Design review of the part built by this model. Coordinates are the model's own, in mm. A direction names the side the tool comes from. Coordinates: 2 decimals unless noted, no trailing zeros. Loops run counter-clockwise (first coordinate to the right, second up) from the corner with the lowest first, then second, coordinate; pieces in that order, holes last. Notation, with made-up numbers: (70.25, -22.75) -> (125.25, -22.75) arc R16 cw to (125.25, -10.75) -> close; hole circle Ø11 at (52.5, -7). An arc over 180 degrees is marked (long way). Use a Markdown table: item, result. Add a question column.
Q1. Take a section at B-B on z = -9.5. Write out the cut boundary in (x, y), plus the area to 3 significant figures.
Q2. Take a section at D-D on z = -13. Write out the cut boundary in (x, y).
Q3. For faces 1 (the face through (-5, 6, -32)), 2 (the face through (-10, 5.9, -11.5)), 3 (the face through (-16.1, 11.5, -4)), 4 (the face through (-29.08, 11.49, -2.45)), 5 (the face through (-15, 1, -7)), list the 3-axis set-ups (+Z, -Z, +X, -X, +Y, -Y) from which the entire face can be reached by the end or side of a thin tool; tool diameter is ignored.
Q4. For probe 1 along X at (y, z) = (11.6, -5); probe 2 along Y at (x, z) = (-17.5, -8); probe 3 along Z at (x, y) = (-26, 0.5), list the stretches that pass through material, from the lowest coordinate up.
Q5. Clearance check with flat-ended pins moving along their axes: pin 1 Ø2 at (x, z) = (-7.5, -7) entering from -Y; pin 2 Ø0.5 at (y, z) = (7.5, -11.5) entering from -X; pin 3 Ø3 at (x, z) = (-26, -5) entering from -Y; pin 4 Ø1 at (y, z) = (4.5, -27) entering from +X. State where each tip first meets the part, or that it passes through.
Q6. Take a section at C-C on x = -15.5. Write out the cut boundary in (y, z), plus the area to 3 significant figures.
Q7. Draft analysis for pull direction Z (two halves, no side actions). For faces 6 (the face through (-16.1, 0.5, -4)), 7 (the face through (-17.888, 11.493, -10.014)), 8 (the face through (-27.6, 11.5, -6.2)), state which applies: pulls with the +Z half, pulls with the -Z half, needs draft (parallel to the pull), parting line crosses it, or undercut.
Q8. Take a section at A-A on x = -5. Write out the cut boundary in (y, z), plus the area to 3 significant figures.
Autodesk Inventor part; units mm, degrees
ref_plane "YZ Plane" through (0, 0, 0) normal (1, 0, 0) x (0, 1, 0)
ref_plane "XZ Plane" through (0, 0, 0) normal (0, 1, 0) x (-1, 0, 0)
ref_plane "XY Plane" through (0, 0, 0) normal (0, 0, 1) x (1, 0, 0)
sketch "Sketch1" plane through (0, 0, 0) normal (0, 1, 0) x (-1, 0, 0)
  line L0 (0, -12) -> (10, -12)
  line L1 (10, -12) -> (10, -5)
  line L2 (0, -5) -> (0, -12)
  arc A0 (10, -5) -> (0, -5) centre (5, -5) ccw
  circle A1 centre (5, -5) radius 2
  circle A2 centre (26, -5) radius 2
  line L3 (10, -4) -> (22, -4)
  line L4 (10, -12) -> (10, -11)
  line L5 (26, -9) -> (10, -11)
  arc A3 (26, -9) -> (22, -5) centre (26, -5) ccw
  line L6 (10, -4) -> (9.899, -4)
  line L7 (22, -4) -> (22.127, -4)
  point P0 (0, 0)
  point P1 (0, 0)
  point P2 (9.9495, -4)
  point P3 (5, 0)
  dimension "d269" = 4
  dimension "d270" = 12
  dimension "d271" = 1
  dimension "d272" = 4
  dimension "d273" = 4
  dimension "d274" = -1
  dimension "d275" = -1
  dimension "d278" = 7
  dimension "d279" = 10
  dimension "d280" = 5
  dimension "d282" = 4
  dimension "d284" = 5
  dimension "d286" = 5
  dimension "d287" = 4
extrude "Extrusion1" add sketch "Sketch1" along normal blind 1
sketch "Sketch2" plane through (0, 1, 0) normal (0, 1, 0) x (1, 0, 0)
  line L0 (0, 12) -> (-10, 12)
  line L1 (0, 12) -> (-10, 12)
  line L2 (-10, 12) -> (-10, 11)
  line L3 (-10, 11) -> (0, 11)
  line L4 (0, 11) -> (0, 12)
  point P0 (0, 0)
  dimension "d288" = 1
extrude "Extrusion2" add sketch "Sketch2" along normal blind 10
sketch "Sketch3" plane through (0, 11, 0) normal (0, 1, 0) x (1, 0, 0)
  line L0 (0, 5) -> (0, 12)
  line L1 (0, 12) -> (-10, 12)
  line L2 (-10, 12) -> (-10, 11)
  line L3 (0, 11) -> (0, 12)
  arc A0 (-9.899, 4) -> (0, 5) centre (-5, 5) ccw
  line L4 (0, 11) -> (0, 5)
  line L5 (-22.127, 4) -> (-9.899, 4)
  arc A1 (-9.899, 4) -> (0, 5) centre (-5, 5) ccw
  arc A2 (-26, 9) -> (-22.127, 4) centre (-26, 5) ccw
  line L6 (-9.899, 4) -> (-22.127, 4)
  line L7 (-10, 11) -> (-26, 9)
  line L8 (-10, 11) -> (-26, 9)
  circle A3 centre (-5, 5) radius 2
  circle A4 centre (-26, 5) radius 2
  arc A5 (-26, 9) -> (-22.127, 4) centre (-26, 5) ccw
  dimension "d291" = 4
  dimension "d294" = 4
  dimension "d295" = 4
extrude "Extrusion3" add sketch "Sketch3" along normal blind 1
sketch "Sketch4" plane through (0, 0, -12) normal (0, 0, -1) x (-1, 0, 0)
  circle A0 centre (5, 6) radius 2
  line L0 (0, 0) -> (10, 0)
  line L1 (0, 0) -> (0, 12)
  dimension "d269" = 4
  dimension "d270" = 12
  dimension "d271" = 1
  dimension "d272" = 4
  dimension "d273" = 4
  dimension "d274" = -1
  dimension "d275" = -1
  dimension "d278" = 7
  dimension "d279" = 10
  dimension "d280" = 5
  dimension "d282" = 4
  dimension "d284" = 5
  dimension "d286" = 5
  dimension "d287" = 4
  dimension "d296" = 4
  dimension "d297" = 6
  dimension "d298" = 5
extrude "Extrusion4" add sketch "Sketch4" along normal blind 20
properties part number "Langbektang houder"
Answer list:
| question | item | result |
|---|---|---|
| 1 | outline | (-22, 0) -> (0, 0) -> (0, 1) -> (-22, 1) -> close; (-22, 11) -> (0, 11) -> (0, 12) -> (-22, 12) -> close |
| 1 | area | 44.0 mm² |
| 2 | outline | circle Ø4 at (-5, 6) |
| 3 | face 1 | -Z, +X, -X, +Y, -Y |
| 3 | face 2 | -Z, -X, +Y, -Y |
| 3 | face 3 | +Z, +Y, -Y |
| 3 | face 4 | +Y, -Y |
| 3 | face 5 | +Z, +X, -X |
| 4 | probe 1 | -30 to -28, -24 to -7, -3 to 0 |
| 4 | probe 2 | 0 to 1, 11 to 12 |
| 4 | probe 3 | -9 to -7, -3 to -1 |
| 5 | pin 1 | y = 0 |
| 5 | pin 2 | x = -10 |
| 5 | pin 3 | through |
| 5 | pin 4 | x = -3.27 |
| 6 | outline | (0, -10.31) -> (1, -10.31) -> (1, -4) -> (0, -4) -> close; (11, -10.31) -> (12, -10.31) -> (12, -4) -> (11, -4) -> close |
| 6 | area | 12.6 mm² |
| 7 | face 6 | pulls with the +Z half |
| 7 | face 7 | pulls with the -Z half |
| 7 | face 8 | undercut |
| 8 | outline | (0, -12) -> (4, -12) -> (4, -32) -> (8, -32) -> (8, -12) -> (12, -12) -> (12, -7) -> (11, -7) -> (11, -11) -> (1, -11) -> (1, -7) -> (0, -7) -> close; (0, -3) -> (1, -3) -> (1, 0) -> (0, 0) -> close; (11, -3) -> (12, -3) -> (12, 0) -> (11, 0) -> close |
| 8 | area | 106 mm² |
